Part model, mm, in its own coordinate system. Give positions to 0.01 mm unless a question says otherwise; leave off trailing zeros. Write each loop counter-clockwise with the first axis right and the second up, starting at its lowest first coordinate (ties: lowest second). Pieces come first, ordered by that corner, then holes. Notation, with made-up numbers: M 6.25,20 L 21.25,20 A28 cw 21.25,40 Z; hole C 61.5,69.25 d5. An arc over 180 degrees is marked long. Answer as CSV lines item,"result". Start each with the question number.
Item 1: Wall check: L1, parallel to X at y = -20.5, z = 22; L2, parallel to X at y = -45.5, z = 19; L3, parallel to Z at x = 5.5, y = -18.5. Give the ranges that are in metal, low to high. Write a range as from..to.
Item 2: Band-saw the part on C-C, the plane y = -5. List the corners of the cut face in (x, z).
Item 3: Band-saw the part on B-B, the plane z = 4.5. List the corners of the cut face in (x, y), then the cut area to 3 significant figures.
Item 4: Pin check, flat tips, straight feed: pin 1 (10 mm diameter, centred on x = 10.5, z = 25.5, fed in from +Y); pin 2 (2 mm diameter, centred on y = -14, z = 25.5, fed in from +X); pin 3 (12 mm diameter, centred on y = -8, z = 32, fed in from +X). Stop position of each tip, or through.
Item 5: Band-saw the part on A-A, the plane y = -31. List the corners of the cut face in (x, z) (3 decimals).
from build123d import *

# Parameters (mm, degrees)
F1_DEPTH      = 50.8
F2_R          = 6.35
F4_DEPTH      = 68.834
F4_DEPTH_BACK = 105


# Not quite as in the source:
# - an extrude ends at something that could not be found from the text; its depth is read off the source's solid


with BuildPart() as f1:
    # F0 (on Front) → F1 (new body)
    with BuildSketch(Plane.XZ):
        Polygon((-25.4, 0), (0, 0), (25.4, 0), (0, 43.9940905122), align=None)
    extrude(amount=F1_DEPTH)

    # F2
    f2_edges = [f1.edges().sort_by_distance(p)[0] for p in [
        (0, -25.4, 43.994091),
        (12.7, -50.8, 21.997045),
        (-12.7, -50.8, 21.997045),
        (0, -50.8, 0),
        (25.4, -25.4, 0),
        (12.7, 0, 21.997045),
        (0, 0, 0),
        (-12.7, 0, 21.997045),
        (-25.4, -25.4, 0),
    ]]
    fillet(f2_edges, radius=F2_R)

    # F3 (on face) → F4 (cut, two sides)
    with BuildSketch(Plane.XZ.offset(50.8)) as f4_sk:
        with BuildLine():
            ThreePointArc((0, 6.35), (5.8793785172, 8.7853183202), (8.3146968374, 14.6646968374))
            ThreePointArc((8.3146968374, 14.6646968374), (8.0313803879, 16.8166988268), (7.200738589, 18.822045424))
            ThreePointArc((7.200738589, 18.822045424), (-9.37e-08, 22.9793936748), (-7.2007386828, 18.8220452616))
            ThreePointArc((-7.2007386828, 18.8220452616), (-7.2007386876, 10.5073484215), (0, 6.35))
        make_face()
    extrude(amount=-F4_DEPTH, mode=Mode.SUBTRACT)
    extrude(f4_sk.sketch, amount=F4_DEPTH_BACK, mode=Mode.SUBTRACT)


solid = f1.part
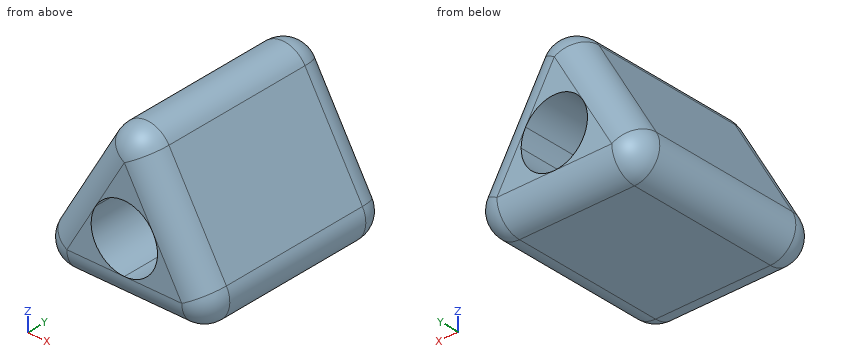
Output:
1,L1,"-12.7..-3.92, 3.92..12.7"
1,L2,"-14.33..-7.1, 7.1..14.33"
1,L3,"0..8.43, 20.9..34.47"
2,outline,"M -19.78,9.45 A6.2 ccw -14.4,0.15 L 14.4,0.15 A6.2 ccw 19.78,9.45 L 5.37,34.4 A6.2 ccw -5.37,34.4 Z; hole C 0,14.66 d16.63"
3,outline,"M -20.48,-44.45 A6.07 ccw -14.4,-50.52 L 14.4,-50.52 A6.07 ccw 20.48,-44.45 L 20.48,-6.35 A6.07 ccw 14.4,-0.28 L -14.4,-0.28 A6.07 ccw -20.48,-6.35 Z"
3,area,"2,030 mm²"
4,pin 1,"y = -0.11"
4,pin 2,"x = 11.25"
4,pin 3,"x = 10.39"
5,outline,"M -19.901,9.525 A6.35 ccw -14.401,0 L 14.401,0 A6.35 ccw 19.901,9.525 L 5.499,34.469 A6.35 ccw -5.499,34.469 Z; hole C 0,14.665 d16.629"
